Print and shaded views of the part. All mm, measured from the part's lowest x, y and z. A direction names the side the tool comes from. Coordinates: 2 decimals unless noted, no trailing zeros. Loops run counter-clockwise (first coordinate to the right, second up) from the corner with the lowest first, then second, coordinate; pieces in that order, holes last. Notation, with made-up numbers: M 30,47 L 85,47 A22 ccw 85,78 Z; hole C 38,40.5 d5. An arc over 180 degrees is marked long. Use a Markdown table: item, result. Add a question column.
1) Band-saw the part on C-C (y = 8.5). List the corners of the cut face in (x, z) (3 decimals), plus the area to 3 significant figures.
2) Band-saw the part on B-B (z = 85.5). List the corners of the cut face in (x, y) (3 decimals), plus the area to 3 significant figures.
3) Wall check: probe 1 along X at (y, z) = (15.5, 50.5) (3 decimals); probe 2 along Z at (x, y) = (38.1, 27.05) (3 decimals); probe 3 along Z at (x, y) = (38.1, 26.4) (3 decimals). Give the ranges that are in metal, low to high. Write a range as from..to.
4) Pull direction X, two halves, no side cores. Call the marked faces 1, 2, 3 and 4: released by +X, released by -X, zero draft, split by the parting line, or undercut.
5) Pin check, flat tips, straight feed: pin 1 Ø5 at (x, z) = (38, 66) entering from -Y; pin 2 Ø6 at (x, y) = (16, 14) entering from +Z (3 decimals); pin 3 Ø7.5 at (y, z) = (9.5, 77.5) entering from -X. Stop position of each tip, or through.
6) Tool access for the marked faces 5, 6 and 7: list every direction of +Z, -Z, +X, -X, +Y, -Y with a clear straight run to the whole face (end or side of a thin tool).
7) Band-saw the part on D-D (x = 38.1). List the corners of the cut face in (y, z) (3 decimals), plus the area to 3 significant figures.
8) Band-saw the part on A-A (x = 69.85). List the corners of the cut face in (y, z) (3 decimals), plus the area to 3 significant figures.
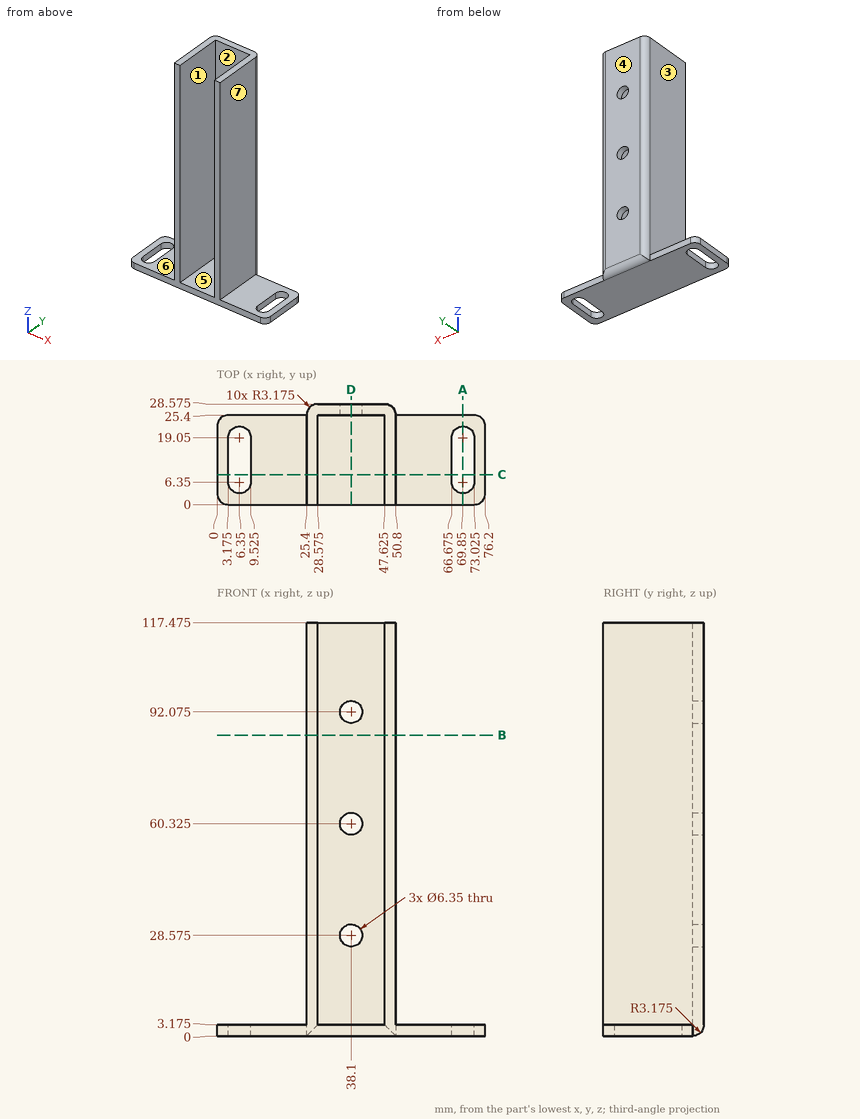
Entries:
| question | item | result |
|---|---|---|
| 1 | outline | M 0,0 L 3.175,0 L 3.175,3.175 L 0,3.175 Z; M 9.525,0 L 66.675,0 L 66.675,3.175 L 50.8,3.175 L 50.8,117.475 L 47.625,117.475 L 47.625,3.175 L 28.575,3.175 L 28.575,117.475 L 25.4,117.475 L 25.4,3.175 L 9.525,3.175 Z; M 73.025,0 L 76.2,0 L 76.2,3.175 L 73.025,3.175 Z |
| 1 | area | 927 mm2 |
| 2 | outline | M 25.4,0 L 28.575,0 L 28.575,25.4 L 47.625,25.4 L 47.625,0 L 50.8,0 L 50.8,25.4 A3.175 ccw 47.625,28.575 L 28.575,28.575 A3.175 ccw 25.4,25.4 Z |
| 2 | area | 238 mm2 |
| 3 | probe 1 | 25.4..28.575, 47.625..50.8 |
| 3 | probe 2 | 0.462..25.4, 31.75..57.15, 63.5..88.9, 95.25..117.475 |
| 3 | probe 3 | 0.162..25.4, 31.75..57.15, 63.5..88.9, 95.25..117.475 |
| 4 | face 1 | undercut |
| 4 | face 2 | undercut |
| 4 | face 3 | released by -X |
| 4 | face 4 | zero draft |
| 5 | pin 1 | y = 25.4 |
| 5 | pin 2 | z = 3.175 |
| 5 | pin 3 | x = 25.4 |
| 6 | face 5 | +Z, -Y |
| 6 | face 6 | +Z, -X, +Y, -Y |
| 6 | face 7 | +Z, +X, +Y, -Y |
| 7 | outline | M 0,0 L 25.4,0 A3.175 ccw 28.575,3.175 L 28.575,25.4 L 25.4,25.4 L 25.4,3.175 L 0,3.175 Z; M 25.4,31.75 L 28.575,31.75 L 28.575,57.15 L 25.4,57.15 Z; M 25.4,63.5 L 28.575,63.5 L 28.575,88.9 L 25.4,88.9 Z; M 25.4,95.25 L 28.575,95.25 L 28.575,117.475 L 25.4,117.475 Z |
| 7 | area | 391 mm2 |
| 8 | outline | M 0,0 L 3.175,0 L 3.175,3.175 L 0,3.175 Z; M 22.225,0 L 25.4,0 L 25.4,3.175 L 22.225,3.175 Z |
| 8 | area | 20.2 mm2 |
